Design review of the part shown in the three views and the two pictorial views. Dimensions are in mm from the part's minimum x, y and z. A direction names the side the tool comes from. Give positions to 0.01 mm unless a question says otherwise; leave off trailing zeros. Order: outer loops, then holes, each group sorted by start corner. A loop starts at its lowest first (then second) coordinate and runs counter-clockwise, first axis right, second up. Notation, with made-up numbers: M 89.25,71.5 L 145.25,71.5 A21 ccw 145.25,110.5 Z; hole C 21.25,-38 d7. An arc over 180 degrees is marked long. Answer as a JSON object with one key per item and string values.
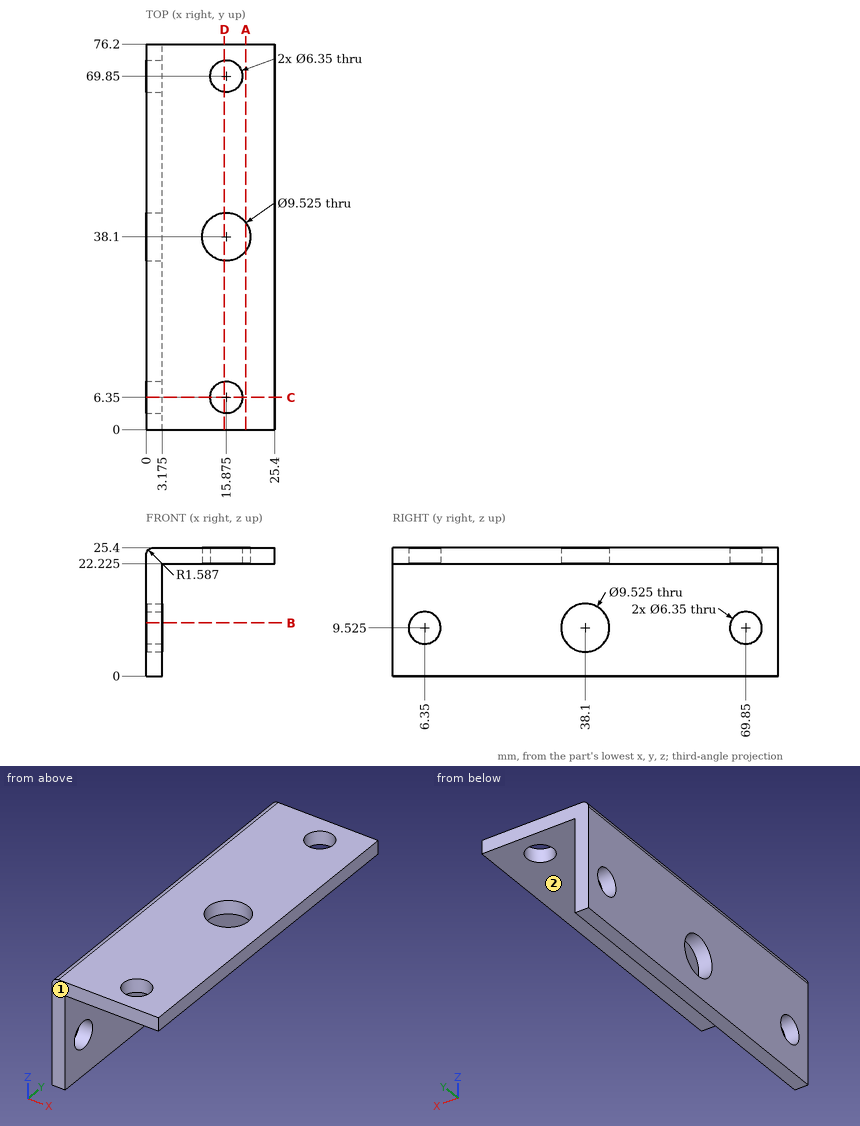
(1) To check wall thickness, follow L1, parallel to Z at x = 1.8, y = 69.85; L2, parallel to X at y = 38, z = 23.25; L3, parallel to Z at x = 22.25, y = 43.5 (1 decimal). State the ranges of each line that lie inside material, in increasing order. Write a range as from..to.
Checked values:
{"L1": "z = 0..6.35, 12.7..25.4", "L2": "x = 0..11.11, 20.64..25.4", "L3": "z = 22.2..25.4"}
(2) We need section C-C (y = 6.35). Count the separate pieces of the cut face and the enclosed holes in it, plus the area to 3 significant figures.
Checked values:
{"separate pieces": "3", "enclosed holes": "0", "area": "110 mm^2"}
(3) We need section B-B (z = 10.5). Write out the cut boundary in (x, y) (1 decimal), plus the area to 3 significant figures.
Checked values:
{"outline": "M 0,0 L 3.2,0 L 3.2,3.3 L 0,3.3 Z; M 0,9.4 L 3.2,9.4 L 3.2,33.4 L 0,33.4 Z; M 0,42.8 L 3.2,42.8 L 3.2,66.8 L 0,66.8 Z; M 0,72.9 L 3.2,72.9 L 3.2,76.2 L 0,76.2 Z", "area": "174 mm^2"}
(4) We need section D-D (x = 15.5). Write out the cut boundary in (y, z) (1 decimal), plus the area to 3 significant figures.
Checked values:
{"outline": "M 0,22.2 L 3.2,22.2 L 3.2,25.4 L 0,25.4 Z; M 9.5,22.2 L 33.4,22.2 L 33.4,25.4 L 9.5,25.4 Z; M 42.8,22.2 L 66.7,22.2 L 66.7,25.4 L 42.8,25.4 Z; M 73,22.2 L 76.2,22.2 L 76.2,25.4 L 73,25.4 Z", "area": "172 mm^2"}
(5) Insertion check: pin 1 (12 mm diameter, centred on x = 20, y = 41, fed in from -Z) (1 decimal); pin 2 (5.5 mm diameter, centred on y = 38.1, z = 9.525, fed in from +X); pin 3 (2 mm diameter, centred on y = 33.5, z = 21, fed in from +X) (1 decimal). Each pin has a flat end and moves straight along its axis. Give the tip position at first contact, or say it passes through.
Checked values:
{"pin 1": "stops at z = 22.2", "pin 2": "passes through", "pin 3": "stops at x = 3.2"}
(6) We need section A-A (x = 19.75). Write out the cut boundary in (y, z) (1 decimal).
Checked values:
{"outline": "M 0,22.2 L 35.3,22.2 L 35.3,25.4 L 0,25.4 Z; M 40.9,22.2 L 76.2,22.2 L 76.2,25.4 L 40.9,25.4 Z"}
(7) Tool access review of the marked faces 1 and 2: name each direction out of +Z, -Z, +X, -X, +Y, -Y from which nothing blocks a thin tool from reaching the whole face with its end or side.
Checked values:
{"face 1": "+Z, -Z, +X, -X, -Y", "face 2": "-Z, +X, +Y, -Y"}
